from build123d import *

# Parameters (mm, degrees)
SKETCH2_W           = 74.422
SKETCH2_H           = 20.574
BOSS_EXTRUDE3_DEPTH = 14.732
SKETCH7_W           = 10.16
SKETCH7_H           = 15.494
BOSS_EXTRUDE4_DEPTH = 11.684
BOSS_EXTRUDE5_DEPTH = 1.016


with BuildPart() as part:
    # Sketch2 → Boss-Extrude3 (new body)
    with BuildSketch(Plane(origin=(0, 0, 0), x_dir=(1, 0, 0), z_dir=(0, 1, 0))):
        with Locations((-2.667, 35.687)):
            Rectangle(SKETCH2_W, SKETCH2_H)
    extrude(amount=BOSS_EXTRUDE3_DEPTH)



with BuildPart() as body_2:
    # Sketch7 → Boss-Extrude4 (new body)
    with BuildSketch(Plane(origin=(0, 0, 0), x_dir=(1, 0, 0), z_dir=(0, 1, 0))):
        with Locations((42.418, 38.227)):
            Rectangle(SKETCH7_W, SKETCH7_H)
    extrude(amount=BOSS_EXTRUDE4_DEPTH)


with BuildPart() as part_1:
    add(part.part)

    add(body_2.part)  # Boss-Extrude5 merges body 2
    # Sketch9 → Boss-Extrude5 (add)
    with BuildSketch(Plane(origin=(0, 0, 0), x_dir=(1, 0, 0), z_dir=(0, 1, 0))):
        with BuildLine():
            Line((-39.878, 43.18), (-52.07, 43.18))
            Line((-52.07, 43.18), (-52.07, 30.48))
            ThreePointArc((-52.07, 30.48), (-49.53, 27.94), (-52.07, 25.4))
            Line((-52.07, 25.4), (-52.07, -43.18))
            Line((-52.07, -43.18), (52.07, -43.18))
            Line((52.07, -43.18), (52.07, 25.4))
            ThreePointArc((52.07, 25.4), (49.53, 27.94), (52.07, 30.48))
            Line((52.07, 30.48), (52.07, 43.18))
            Line((52.07, 43.18), (47.498, 43.18))
            Line((47.498, 43.18), (47.498, 30.48))
            Line((47.498, 30.48), (37.338, 30.48))
            Line((37.338, 30.48), (37.338, 43.18))
            Line((37.338, 43.18), (34.544, 43.18))
            Line((34.544, 43.18), (34.544, 25.4))
            Line((34.544, 25.4), (-39.878, 25.4))
            Line((-39.878, 25.4), (-39.878, 43.18))
        make_face()
    extrude(amount=BOSS_EXTRUDE5_DEPTH)


solid = part_1.part
The listing builds one solid part. Answer for the finished solid, in the listing's coordinates (mm). A direction names the side the tool comes from. Round coordinates to 2 decimals unless told otherwise and drop trailing zeros. Order: outer loops, then holes, each group sorted by start corner. A loop starts at its lowest first (then second) coordinate and runs counter-clockwise, first axis right, second up. Notation, with made-up numbers: (45, 43) -> (56, 43) arc R28 ccw to (56, 64) -> close; hole circle Ø10 at (88, 1.5). An arc over 180 degrees is marked (long way). Put each result on its own line as item: value.
Q1. Each of these flat-tipped pins is pushed along its axis until it touches: P1, Ø0.5, axis at x = -44.5, y = 0.5, coming from the -Z side; P2, Ø5, axis at x = 40, z = -34.5, coming from the +Y side; P3, Ø7.5, axis at y = 6.5, z = -37, coming from the -X side. Where does it stop, or does it pass through?
Results list:
P1: z = -43.18
P2: y = 11.68
P3: x = -39.88
Q2. Determine the mould class of faces 1 (the flat face through (34.544, 7, -36)), 2 (the flat face through (-3, 14.732, -36)), 3 (the cylindrical face through (49.53, 0.5, -27.88)) for opening direction X: pulls with the +X half, pulls with the -X half, needs draft (parallel to the pull), parting line crosses it, or undercut.
Results list:
face 1: undercut
face 2: needs draft
face 3: pulls with the +X half
Q3. Section D-D, the plane x = 44.5 is taken. Write down the section's boundary in (y, z), and give its area (3 significant figures).
Results list:
outline: (0, -45.97) -> (11.68, -45.97) -> (11.68, -30.48) -> (1.02, -30.48) -> (1.02, 43.18) -> (0, 43.18) -> close
area: 256 mm^2
Q4. Which of the six approach directions +Z, -Z, +X, -X, +Y, -Y give full straight-line access (tool end or side, diameter ignored) to faces 4 (the flat face through (42, 11.684, -38)), 5 (the flat face through (42, 6, -30.48)), 6 (the flat face through (-3, 8, -25.4))?
Results list:
face 4: +Z, -Z, +X, +Y
face 5: +Z, +X, +Y
face 6: +Z, +X, -X, +Y
Q5. Section B-B, the plane z = -35.5 is taken. Write down the section's boundary in (x, y), and give its area (3 significant figures).
Results list:
outline: (-52.07, 0) -> (52.07, 0) -> (52.07, 1.02) -> (47.5, 1.02) -> (47.5, 11.68) -> (37.34, 11.68) -> (37.34, 1.02) -> (34.54, 1.02) -> (34.54, 14.73) -> (-39.88, 14.73) -> (-39.88, 1.02) -> (-52.07, 1.02) -> close
area: 1,230 mm^2
Q6. Section A-A, the plane y = 5.75 is taken. Write down the section's boundary in (x, z).
Results list:
outline: (-39.88, -45.97) -> (34.54, -45.97) -> (34.54, -25.4) -> (-39.88, -25.4) -> close; (37.34, -45.97) -> (47.5, -45.97) -> (47.5, -30.48) -> (37.34, -30.48) -> close
Q7. Section C-C, the plane x = -16 is taken. Write down the section's boundary in (y, z), and give its area (3 significant figures).
Results list:
outline: (0, -45.97) -> (14.73, -45.97) -> (14.73, -25.4) -> (1.02, -25.4) -> (1.02, 43.18) -> (0, 43.18) -> close
area: 373 mm^2
Q8. Consider line 1 along Y through (x, z) = (34.5, 25); line 2 along Z through (x, y) = (-13.5, 8.75); line 3 along Z through (x, y) = (40, 10.5). Determine where each line is inside the solid, lowest interval first.
Results list:
line 1: 0 to 1.02
line 2: -45.97 to -25.4
line 3: -45.97 to -30.48
